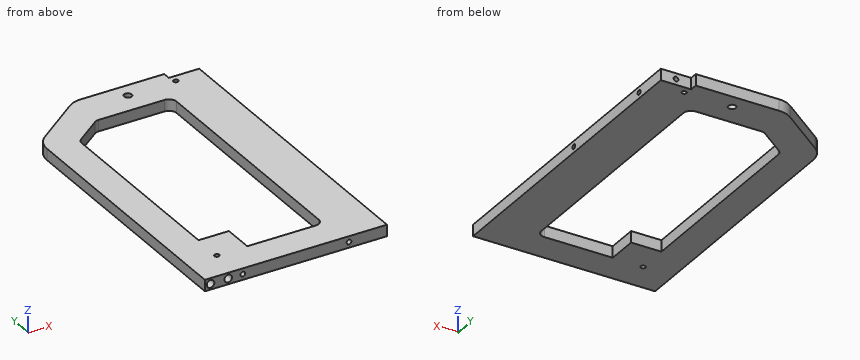
Solid Edge part; units mm, degrees
sketch "Sketch1" plane through (0, 0, 0) normal (0, 0, 1) x (1, 0, 0)
  line L0 (0, 0) -> (0, 266.7)
  line L1 (0, 266.7) -> (152.4, 266.7)
  line L2 (152.4, 266.7) -> (152.4, 0)
  line L3 (152.4, 0) -> (0, 0)
  dimension "D1" = 152.4
extrude "Protrusion1" add sketch "Sketch1" along normal blind 9.525
hole "Hole_1" at (88.9, 254, 9.525) direction (0, 0, -1) diameter 6.35 end through all
sketch "Sketch2" plane through (76.2, 133.35, 9.525) normal (0, 0, 1) x (1, 0, 0)
  line L0 (-76.2, 133.35) -> (-25.4, 133.35)
  line L1 (-25.4, 133.35) -> (-76.2, 95.25)
  line L2 (-76.2, 95.25) -> (-76.2, 133.35)
  dimension "D1" = 76.2
  dimension "D2" = 76.2
extrude "Cutout1" cut sketch "Sketch2" against normal through all
sketch "Sketch3" plane through (38.1, 127, 9.525) normal (0, 0, 1) x (1, 0, 0)
  line L0 (-12.7, 88.9) -> (-12.7, -76.2)
  line L1 (-12.7, -76.2) -> (12.7, -76.2)
  line L2 (12.7, -76.2) -> (12.7, -101.6)
  line L3 (12.7, -101.6) -> (76.2, -101.6)
  line L4 (76.2, -101.6) -> (76.2, 107.95)
  line L5 (76.2, 107.95) -> (12.7, 107.95)
  line L6 (-12.7, 88.9) -> (12.7, 107.95)
  dimension "D1" = 12.7
  dimension "D2" = 12.7
  dimension "D3" = 12.7
extrude "Cutout2" cut sketch "Sketch3" against normal through all
sketch "Sketch4" plane through (44.45, 133.35, 9.525) normal (0, 0, 1) x (1, 0, 0)
  line L0 (107.95, 133.35) -> (107.95, 127)
  line L1 (107.95, 127) -> (82.55, 127)
  line L2 (82.55, 127) -> (82.55, 133.35)
  line L3 (82.55, 133.35) -> (107.95, 133.35)
  dimension "D1" = 107.95
  dimension "D2" = 82.55
extrude "Cutout3" cut sketch "Sketch4" against normal through all
hole "Hole_9" at (120.65, 0, 4.7625) direction (0, 1, 0) diameter 3.9675 depth 19.05
hole "Hole1" at (31.75, 0, 4.7625) direction (0, 1, 0) diameter 3.9675 depth 19.05
hole "Hole_3" at (139.7, 260.35, 4.7625) direction (0, -1, 0) diameter 3.9675 depth 19.05
hole "Hole2" [suppressed]
hole "Hole_4a" at (25.4, 25.4, 9.525) direction (0, 0, -1) diameter 3.9675 end through all
fillet "Round_1" radius 19.05 2 edges at (0, 228.6, 4.7625) (50.8, 266.7, 4.7625)
fillet "Round_2" radius 6.35 4 edges at (50.8, 234.95, 4.7625) (114.3, 234.95, 4.7625) (114.3, 25.4, 4.7625) (25.4, 215.9, 4.7625)
hole "Hole3" at (19.4945, 0, 4.7625) direction (0, 1, 0) diameter 6.35 depth 25.4
hole "Hole4" at (4.7625, 0, 4.7625) direction (0, 1, 0) diameter 6.35 depth 25.4
hole "Hole_16" at (152.4, 230.1875, 4.7625) direction (-1, 0, 0) diameter 3.9675 depth 12.7
hole "Hole5" at (152.4, 139.7, 4.7625) direction (-1, 0, 0) diameter 3.9675 depth 12.7
hole "Hole_18" at (129.032, 254, 9.525) direction (0, 0, -1) diameter 3.9675 end up to next
properties part number "CHAS-02" material "Polyethylene, low density"
Read the model definition and answer for the solid it produces. Units are mm, in the model's axes. Round coordinates to 2 decimals unless told otherwise and drop trailing zeros. Write each loop counter-clockwise with the first axis right and the second up, starting at its lowest first coordinate (ties: lowest second). Pieces come first, ordered by that corner, then holes. Notation, with made-up numbers: (87, 65) - (122, 65) arc R29 ccw to (122, 89) - close; hole circle Ø2 at (15.25, -12). An arc over 180 degrees is marked (long way). Use a Markdown table: item, result.
(1) Straight lines are drawn through the part: line 1 along Y through (x, z) = (76.5, 7); line 2 along Y through (x, z) = (88.9, 6.25) (3 decimals); line 3 along X through (y, z) = (181, 8.5). For each, find the intervals that lie inside material, in ascending order. Write a range as [from, to].
Reported:
| item | result |
|---|---|
| line 1 | [0, 25.4], [234.95, 266.7] |
| line 2 | [0, 25.4], [234.95, 250.825], [257.175, 266.7] |
| line 3 | [0, 25.4], [114.3, 152.4] |
(2) Each of these flat-tipped pins is pushed along its axis until it touches: pin 1 Ø5 at (x, z) = (19.49, 4.76) entering from +Y; pin 2 Ø3 at (x, z) = (5, 3.5) entering from -Y; pin 3 Ø1.2 at (y, z) = (230.5, 5) entering from +X. Where does it stop, or does it pass through?
Reported:
| item | result |
|---|---|
| pin 1 | y = 245.09 |
| pin 2 | y = 25.4 |
| pin 3 | x = 139.7 |
(3) The part is cut by section C-C (z = 4.5). State how many separate pieces and enclosed holes the cut face has, then the cut area to 3 significant figures.
Reported:
| item | result |
|---|---|
| separate pieces | 1 |
| enclosed holes | 4 |
| area | 21,100 mm2 |
(4) The part is cut by section A-A (y = 162). Write down the section's boundary in (x, z) (3 decimals).
Reported:
| item | result |
|---|---|
| outline | (0, 0) - (25.4, 0) - (25.4, 9.525) - (0, 9.525) - close; (114.3, 0) - (152.4, 0) - (152.4, 9.525) - (114.3, 9.525) - close |
(5) The part is cut by section B-B (x = 63). Write down the section's boundary in (y, z) (3 decimals), then the cut area to 3 significant figures.
Reported:
| item | result |
|---|---|
| outline | (0, 0) - (25.4, 0) - (25.4, 9.525) - (0, 9.525) - close; (234.95, 0) - (266.7, 0) - (266.7, 9.525) - (234.95, 9.525) - close |
| area | 544 mm2 |
